from build123d import *

# Parameters (mm, degrees)
SKETCH_1_R          = 1.75
EXTRUDE_1_DEPTH     = 6.6
EXTRUDE_1_2_DEPTH   = 6.6
SKETCH_2_R          = 50
EXTRUDE_2_DEPTH     = 3.4
SKETCH_4_R          = 1.75
CUT_EXTRUDE_2_DEPTH = 10
EXTRUDE_7_DEPTH     = 20
SKETCH_10_W         = 36
SKETCH_10_H         = 48.823085464
CUT_EXTRUDE_3_DEPTH = 10
SKETCH_11_R         = 3
CUT_EXTRUDE_6_DEPTH = 10
EXTRUDE_8_DEPTH     = 4.3


with BuildPart() as part:
    # Sketch 1 → Extrude 1 (new body)
    with BuildSketch(Plane.XY):
        with BuildLine():
            ThreePointArc((20.506096654, 20.506096654), (29, 0), (20.506096654, -20.506096654))
            Line((20.506096654, -20.506096654), (24.748737342, -24.748737342))
            ThreePointArc((24.748737342, -24.748737342), (24.748737342, -35.355339059), (35.355339059, -35.355339059))
            ThreePointArc((35.355339059, -35.355339059), (50, 0), (35.355339059, 35.355339059))
            ThreePointArc((35.355339059, 35.355339059), (24.748737342, 35.355339059), (24.748737342, 24.748737342))
            Line((24.748737342, 24.748737342), (20.506096654, 20.506096654))
        make_face()
        with Locations((30.0520382, 30.0520382)):
            Circle(SKETCH_1_R, mode=Mode.SUBTRACT)
        with Locations((30.0520382, -30.0520382)):
            Circle(SKETCH_1_R, mode=Mode.SUBTRACT)
        with Locations((42.5, 0)):
            Circle(SKETCH_1_R, mode=Mode.SUBTRACT)
    extrude(amount=EXTRUDE_1_DEPTH)



with BuildPart() as body_2:
    # Sketch 1 → Extrude 1 2 (new body)
    with BuildSketch(Plane.XY):
        with BuildLine():
            ThreePointArc((-35.355339059, 35.355339059), (-50, 0), (-35.355339059, -35.355339059))
            ThreePointArc((-35.355339059, -35.355339059), (-24.748737342, -35.355339059), (-24.748737342, -24.748737342))
            Line((-24.748737342, -24.748737342), (-20.506096654, -20.506096654))
            ThreePointArc((-20.506096654, -20.506096654), (-29, 0), (-20.506096654, 20.506096654))
            Line((-20.506096654, 20.506096654), (-24.748737342, 24.748737342))
            ThreePointArc((-24.748737342, 24.748737342), (-24.748737342, 35.355339059), (-35.355339059, 35.355339059))
        make_face()
        with Locations((-30.0520382, 30.0520382)):
            Circle(SKETCH_1_R, mode=Mode.SUBTRACT)
        with Locations((-30.0520382, -30.0520382)):
            Circle(SKETCH_1_R, mode=Mode.SUBTRACT)
        with Locations((-42.5, 0)):
            Circle(SKETCH_1_R, mode=Mode.SUBTRACT)
    extrude(amount=EXTRUDE_1_2_DEPTH)


with BuildPart() as part_1:
    add(part.part)

    add(body_2.part)  # Extrude 2 merges body 2
    # Sketch 2 → Extrude 2 (add)
    with BuildSketch(Plane.XY.offset(6.6)):
        with Locations(Location((0, 0, 0), (0, 0, 225))):
            Circle(SKETCH_2_R)
    extrude(amount=EXTRUDE_2_DEPTH)

    # Sketch 4 → Cut-Extrude 2 (cut, symmetric)
    with BuildSketch(Plane(origin=(0, 0, 6.6), x_dir=(-1, 0, 0), z_dir=(0, 0, -1))):
        with Locations(Location((-42.5, 0, 0), (0, 0, 180))):
            Circle(SKETCH_4_R)
        with Locations(Location((-30.0520382, 30.0520382, 0), (0, 0, 180))):
            Circle(SKETCH_4_R)
        with Locations(Location((-30.0520382, -30.0520382, 0), (0, 0, 180))):
            Circle(SKETCH_4_R)
        with Locations(Location((30.0520382, -30.0520382, 0), (0, 0, 180))):
            Circle(SKETCH_4_R)
        with Locations(Location((42.5, 0, 0), (0, 0, 180))):
            Circle(SKETCH_4_R)
        with Locations(Location((30.0520382, 30.0520382, 0), (0, 0, 180))):
            Circle(SKETCH_4_R)
    extrude(amount=CUT_EXTRUDE_2_DEPTH, both=True, mode=Mode.SUBTRACT)

    # Sketch 5 → Extrude 7 (add)
    with BuildSketch(Plane.XY.offset(10)):
        Polygon((-18, -31.176914536), (-18, -80), (18, -80), (18, -31.176914536), (36, 0), (18, 31.176914536), (18, 80), (-18, 80), (-18, 31.176914536), (-36, 0), align=None)
    extrude(amount=EXTRUDE_7_DEPTH)

    # Sketch 10 → Cut-Extrude 3 (cut)
    with BuildSketch(Plane.XY.offset(30)):
        with Locations((0, -55.588457268)):
            Rectangle(SKETCH_10_W, SKETCH_10_H)
        with Locations((0, 55.588457268)):
            Rectangle(SKETCH_10_W, SKETCH_10_H)
    extrude(amount=-CUT_EXTRUDE_3_DEPTH, mode=Mode.SUBTRACT)

    # Sketch 11 → Cut-Extrude 6 (cut)
    with BuildSketch(Plane.XY.offset(20)):
        with Locations((0, 62)):
            Circle(SKETCH_11_R)
    cut_extrude_6 = extrude(amount=-CUT_EXTRUDE_6_DEPTH, mode=Mode.SUBTRACT)

    # Mirror 2: Cut-Extrude 6 across plane
    add(cut_extrude_6.mirror(Plane.ZX), mode=Mode.SUBTRACT)

    # Sketch 12 → Extrude 8 (add)
    with BuildSketch(Plane.XY.offset(30)):
        Polygon((36, 0), (18, 31.176914536), (-18, 31.176914536), (-36, 0), (-18, -31.176914536), (18, -31.176914536), align=None)
    extrude(amount=EXTRUDE_8_DEPTH)


solid = part_1.part
Input: part model. Units: mm. Frame: model coordinates. A direction names the side the tool comes from. Give positions to 0.01 mm unless a question says otherwise; leave off trailing zeros. Write each loop counter-clockwise with the first axis right and the second up, starting at its lowest first coordinate (ties: lowest second). Pieces come first, ordered by that corner, then holes. Notation, with made-up numbers: M -8,-32 L 5,-32 A15 ccw 5,-19 Z; hole C 50.5,-7.75 d9. An arc over 180 degrees is marked long. Write item = value, one per line. Start each with the question number.
1) Cut plane B-B on x = 0. Return the cut outline in (y, z).
2) Reachability of faces 1 (the flat face through (26.87, -15.81, 21.98)), 2 (the flat face through (27.126, 15.37, 21.98)), 3 (the flat face through (0, -55, 20)), 4 (the cylindrical face through (24.9, 35.5, 3.3)), 5 (the flat face through (-26.87, 15.81, 21.98)) from +Z, -Z, +X, -X, +Y, -Y: full face, straight path, thin tool, end or side. Return the list, or none.
3) Cut plane D-D on z = 3. Return the cut outline in (x, y).
4) First-contact query: pin 1 Ø12 at (x, z) = (-35.5, 4) entering from +Y; pin 2 Ø3 at (x, y) = (-30.05, -30.05) entering from +Z; pin 3 Ø11 at (y, z) = (61.5, 16) entering from +X; pin 4 Ø8 at (x, z) = (-39, 7.5) entering from -Y. Flat tips, straight axial feed; report the tip coordinate or a pass-through.
5) Cut plane A-A on z = 18. Return the cut outline in (x, y), then the cut area to 3 significant figures.
6) Cut plane C-C on y = 62. Return the cut outline in (x, z), then the cut area to 3 significant figures.
7) Material intervals for line 1 along Y through (x, z) = (0, 16); line 2 along X through (y, z) = (0, 6.5); line 3 along X through (y, z) = (-62, 12.5), sorted ascending. Write a range as [from, to].
8) Draft query along X for faces 6 (the flat face through (-18, -55, 15)), 7 (the cylindrical face through (29, 0, 3)), 8 (the cylindrical face through (-24.9, -35.5, 3.3)), 9 (the flat face through (35, 1, 0)). Return one class per face: +X half, -X half, draft (parallel to the pull), parting line (faces both ways), or undercut.
Solved:
q1.outline = M -80,10 L -65,10 L -65,20 L -80,20 Z; M -59,10 L -50,10 L -50,6.6 L 50,6.6 L 50,10 L 59,10 L 59,20 L 31.18,20 L 31.18,34.3 L -31.18,34.3 L -31.18,20 L -59,20 Z; M 65,10 L 80,10 L 80,20 L 65,20 Z
q2.face_1 = +Z, +X, -Y
q2.face_2 = +Z, +X, +Y
q2.face_3 = +Z, +X, -X, -Y
q2.face_4 = -Z
q2.face_5 = +Z, -X, +Y
q3.outline = M -35.36,-35.36 A7.5 ccw -24.75,-24.75 L -20.51,-20.51 A29 cw -20.51,20.51 L -24.75,24.75 A7.5 ccw -35.36,35.36 A50 ccw Z; M 20.51,-20.51 L 24.75,-24.75 A7.5 ccw 35.36,-35.36 A50 ccw 35.36,35.36 A7.5 ccw 24.75,24.75 L 20.51,20.51 A29 cw Z; hole C -42.5,0 d3.5; hole C -30.05,-30.05 d3.5; hole C -30.05,30.05 d3.5; hole C 30.05,-30.05 d3.5; hole C 30.05,30.05 d3.5; hole C 42.5,0 d3.5
q4.pin_1 = 39.93
q4.pin_2 = through
q4.pin_3 = 18
q4.pin_4 = -35.71
q5.outline = M -36,0 L -18,-31.18 L -18,-80 L 18,-80 L 18,-31.18 L 36,0 L 18,31.18 L 18,80 L -18,80 L -18,31.18 Z; hole C 0,-62 d6; hole C 0,62 d6
q5.area = 6,830 mm2
q6.outline = M -18,10 L -3,10 L -3,20 L -18,20 Z; M 3,10 L 18,10 L 18,20 L 3,20 Z
q6.area = 300 mm2
q7.line_1 = [-80, -65], [-59, 59], [65, 80]
q7.line_2 = [-50, -44.25], [-40.75, -29], [29, 40.75], [44.25, 50]
q7.line_3 = [-18, -3], [3, 18]
q8.face_6 = -X half
q8.face_7 = undercut
q8.face_8 = undercut
q8.face_9 = draft
